Work out the finished part from the listing and answer in its coordinate system (mm). A direction names the side the tool comes from. Give positions to 0.01 mm unless a question says otherwise; leave off trailing zeros. Loops run counter-clockwise (first coordinate to the right, second up) from the corner with the lowest first, then second, coordinate; pieces in that order, holes last. Notation, with made-up numbers: (70, 63) - (108, 63) arc R11 cw to (108, 79) - close; hole circle Ø8 at (45.5, 36). An arc over 180 degrees is marked (long way). One line per item, written item: value.
from build123d import *

# Parameters (mm, degrees)
F2_DEPTH = 926
F0_R     = 6
F3_DEPTH = 594
F5_DEPTH = 769


with BuildPart() as f2:
    # F1 (on Top) → F2 (new body)
    with BuildSketch(Plane.XY):
        Polygon((0, 700), (0, 0), (20, 0), (20, 680), (420, 680), (420, 35), (410, 35), (410, 5), (420, 5), (420, 0), (440, 0), (440, 5), (520.748317, 5), (520.748317, 35), (440, 35), (440, 700), align=None)
    extrude(amount=F2_DEPTH)

    # F0 (on Right) → F3 (intersect, symmetric)
    with BuildSketch(Plane.YZ):
        Polygon((0, 20), (0, 0), (800, 0), (800, 20), (35, 20), (35, 500), (5, 500), (5, 20), align=None)
        with Locations((100, 10)):
            Circle(F0_R, mode=Mode.SUBTRACT)
        with Locations((20, 480)):
            Circle(F0_R, mode=Mode.SUBTRACT)
    extrude(amount=F3_DEPTH, both=True, mode=Mode.INTERSECT)

    # F4 (on Front) → F5 (intersect)
    with BuildSketch(Plane.XZ):
        Polygon((0, 20), (0, 0), (440, 0), (440, 20), (420, 20), (420, 415), (475, 415), (475, 520), (465, 520), (465, 425), (420, 425), (420, 520), (410, 520), (410, 20), align=None)
    extrude(amount=-F5_DEPTH, mode=Mode.INTERSECT)


solid = f2.part
1. The mould has two halves that part along Y. Classify faces 5 (the flat face through (418, 5, 304)), 6 (the flat face through (420, 20, 462)), 7 (the flat face through (420, 362, 10)): released by +Y, released by -Y, zero draft, split by the parting line, or undercut.
Output:
face 5: released by -Y
face 6: zero draft
face 7: undercut
2. Flat-ended cylindrical pins translate along their axes: pin 1 Ø22 at (y, z) = (477.5, 13) entering from -X; pin 2 Ø6 at (x, z) = (275.5, 7) entering from -Y; pin 3 Ø6 at (y, z) = (452.5, 11) entering from +X; pin 4 Ø9 at (y, z) = (20, 290) entering from -X. Find the tip coordinate at first contact, or state that the pin passes through.
Output:
pin 1: stops at x = 0
pin 2: stops at y = 680
pin 3: stops at x = 440
pin 4: stops at x = 410
3. Section C-C (z = 174) is taken. Write down the section's boundary in (x, y).
Output:
outline: (410, 5) - (420, 5) - (420, 35) - (410, 35) - close
4. Find the intervals of material crossed by line 1 along Z through (x, y) = (14.5, 100); line 2 along Z through (x, y) = (470.5, 20); line 3 along Y through (x, z) = (429, 10), in increasing order.
Output:
line 1: z = 0 to 4, 16 to 20
line 2: z = 415 to 474, 486 to 500
line 3: y = 0 to 94, 106 to 700
5. For faces 1 (the flat face through (447, 20, 415)), 2 (the flat face through (431, 455, 0)), 3 (the flat face through (20, 335, 10)), 4 (the flat face through (443, 20, 425)), determine the directions among +Z, -Z, +X, -X, +Y, -Y from which every point of the face is accessible in a straight line to the end or side of a thin tool.
Output:
face 1: +X, +Y, -Y
face 2: -Z, +X, -X, +Y, -Y
face 3: +Z, -Z, -Y
face 4: +Z, +Y, -Y
6. Section B-B (y = 566) is taken. Write down the section's boundary in (x, z), and give its area (3 significant figures).
Output:
outline: (0, 0) - (20, 0) - (20, 20) - (0, 20) - close; (420, 0) - (440, 0) - (440, 20) - (420, 20) - close
area: 800 mm²
7. Section D-D (x = 362.5) is taken. Write down the section's boundary in (y, z).
Output:
outline: (680, 0) - (700, 0) - (700, 20) - (680, 20) - close
8. Section A-A (z = 441) is taken. Write down the section's boundary in (x, y).
Output:
outline: (410, 5) - (420, 5) - (420, 35) - (410, 35) - close; (465, 5) - (475, 5) - (475, 35) - (465, 35) - close
